For this review, take the finished solid that the model builds, in its own axes (mm). A direction names the side the tool comes from. Coordinates: 2 decimals unless noted, no trailing zeros. Write each loop counter-clockwise with the first axis right and the second up, starting at its lowest first coordinate (ties: lowest second). Pieces come first, ordered by that corner, then holes. Notation, with made-up numbers: M 15.25,68.25 L 66.25,68.25 A24 ccw 66.25,101.25 Z; hole C 18,4.5 d1. An arc over 180 degrees is marked long. One line per question, with ' | ' between items.
from build123d import *

# Parameters (mm, degrees)
SKETCH_1_W             = 20
SKETCH_1_H             = 20
EXTRUDE_1_DEPTH        = 3
SKETCH_2_W             = 20
SKETCH_2_H             = 3
EXTRUDE_2_DEPTH        = 23
HOLE_WIZARD_M3_1_D     = 2.5
HOLE_WIZARD_M3_1_DEPTH = 7.5
HOLE_WIZARD_M3_1_TIP   = 0.751075774
HOLE_WIZARD_M3_2_D     = 2.5
HOLE_WIZARD_M3_2_DEPTH = 7.5
HOLE_WIZARD_M3_2_TIP   = 0.751075774
CHAMFER_1_SIZE         = 1


with BuildPart() as part:
    # 草图1 → 凸台-拉伸1 (new body)
    with BuildSketch(Plane.XY):
        Rectangle(SKETCH_1_W, SKETCH_1_H)
    extrude(amount=EXTRUDE_1_DEPTH)

    # 草图2 → 凸台-拉伸2 (add)
    with BuildSketch(Plane.XY.offset(3)):
        with Locations((0, -11.5)):
            Rectangle(SKETCH_2_W, SKETCH_2_H)
    extrude(amount=-EXTRUDE_2_DEPTH)

    # M3 螺纹孔1
    with Locations(Plane(origin=(0, 0, 0), x_dir=(-1, 0, 0), z_dir=(0, 0, -1))):
        with Locations((5, 5), (-5, -5)):
            Hole(HOLE_WIZARD_M3_1_D / 2, depth=HOLE_WIZARD_M3_1_DEPTH)
            with Locations((0, 0, -(HOLE_WIZARD_M3_1_DEPTH + HOLE_WIZARD_M3_1_TIP / 2))):  # 118° drill point
                Cone(0, HOLE_WIZARD_M3_1_D / 2, HOLE_WIZARD_M3_1_TIP, mode=Mode.SUBTRACT)

    # M3 螺纹孔2
    with Locations(Plane(origin=(0, -10, 0), x_dir=(1, 0, 0), z_dir=(0, 1, 0))):
        with Locations((-5, 15), (5, 5)):
            Hole(HOLE_WIZARD_M3_2_D / 2, depth=HOLE_WIZARD_M3_2_DEPTH)
            with Locations((0, 0, -(HOLE_WIZARD_M3_2_DEPTH + HOLE_WIZARD_M3_2_TIP / 2))):  # 118° drill point
                Cone(0, HOLE_WIZARD_M3_2_D / 2, HOLE_WIZARD_M3_2_TIP, mode=Mode.SUBTRACT)

    # 倒角1
    chamfer_1_edges = [part.edges().sort_by_distance(p)[0] for p in [
        (-10, -11.5, -20),
        (10, -11.5, -20),
        (-10, 10, 1.5),
        (10, 10, 1.5),
    ]]
    chamfer(chamfer_1_edges, length=CHAMFER_1_SIZE)


solid = part.part
1. Take a section at A-A on x = -4.25. State the section outline as (y, z) points, plus the area to 3 significant figures.
Computed values:
outline: M -13,-20 L -10,-20 L -10,-16 L -13,-16 Z; M -13,-14 L -10,-14 L -10,0 L 4,0 L 4,3 L -13,3 Z; M 6,0 L 10,0 L 10,3 L 6,3 Z | area: 117 mm2
2. For line 1 along Z through (x, y) = (5, -10.85); line 2 along X through (y, z) = (-11.25, -15); line 3 along Z through (x, y) = (-5, -10.85), list the stretches that pass through material, from the lowest coordinate up.
Computed values:
line 1: z = -20 to -6.25, -3.75 to 3 | line 2: x = -10 to -6.25, -3.75 to 10 | line 3: z = -20 to -16.25, -13.75 to 3
3. Clearance check with flat-ended pins moving along their axes: P1, Ø10, axis at x = 0.5, y = -4.5, coming from the -Z side; P2, Ø5, axis at y = -5, z = -4.5, coming from the +X side. State where each tip first meets the part, or that it passes through.
Computed values:
P1: stops at z = 0 | P2: passes through
4. Take a section at B-B on z = -15. State the section outline as (x, y) points.
Computed values:
outline: M -10,-13 L -6.25,-13 L -6.25,-10 L -10,-10 Z; M -3.75,-13 L 10,-13 L 10,-10 L -3.75,-10 Z
5. Draft analysis for pull direction Y (two halves, no side actions). For faces 1 (the flat face through (0, 10, 1)), 2 (the cylindrical face through (5.27, -11.52, -3.78)), 3 (the cylindrical face through (-5.27, 3.78, 1.52)), state which applies: pulls with the +Y half, pulls with the -Y half, needs draft (parallel to the pull), parting line crosses it, or undercut.
Computed values:
face 1: pulls with the +Y half | face 2: needs draft | face 3: undercut
6. Machinability: for faces 4 (the flat face through (0, 0, 0)), 5 (the flat face through (-9.5, 9.5, 1.5)), which of the approach directions +Z, -Z, +X, -X, +Y, -Y give a long, thin tool a straight path to every point of the face, cutting with its end or side? Answer none if there is none.
Computed values:
face 4: -Z, +X, -X, +Y | face 5: +Z, -Z, -X, +Y
7. Take a section at C-C on y = 5. State the section outline as (x, z) points, plus the area to 3 significant figures.
Computed values:
outline: M -10,0 L -6.25,0 L -6.25,3 L -10,3 Z; M -3.75,0 L 10,0 L 10,3 L -3.75,3 Z | area: 52.5 mm2
8. Take a section at D-D on x = 5. State the section outline as (y, z) points, plus the area to 3 significant figures.
Computed values:
outline: M -13,-20 L -10,-20 L -10,-6.25 L -13,-6.25 Z; M -13,-3.75 L -10,-3.75 L -10,0 L -6.25,0 L -6.25,3 L -13,3 Z; M -3.75,0 L 10,0 L 10,3 L -3.75,3 Z | area: 114 mm2
